The model under review builds one solid part; all positions refer to its coordinate system, in mm. Give positions to 0.01 mm unless a question says otherwise; leave off trailing zeros. Loops run counter-clockwise (first coordinate to the right, second up) from the corner with the lowest first, then second, coordinate; pieces in that order, holes last. Notation, with made-up numbers: M 20.25,-21 L 68.25,-21 A13 cw 68.25,-4 Z; hole C 77.25,-11.5 d8. An arc over 180 degrees is marked long. Return JSON: item names as keys, results as strings.
```python
from build123d import *

# Parameters (mm, degrees)
SKETCH1_W                      = 3
SKETCH1_H                      = 12.5
BOSS_EXTRUDE1_DEPTH            = 668
SKETCH2_R                      = 2
CUT_EXTRUDE1_DEPTH             = 10
CHAMFER1_SIZE                  = 2.5
LPATTERN1_COUNT                = 14
LPATTERN1_PITCH                = 50
CHAMFER1_OF_LPATTERN1_SIZE     = 2.5
LPATTERN1_COL_COUNT            = 14
LPATTERN1_COL_PITCH            = 50
CHAMFER1_OF_LPATTERN1_COL_SIZE = 2.5
CHAMFER2_SIZE                  = 1


with BuildPart() as part:
    # Sketch1 → Boss-Extrude1 (new, symmetric)
    with BuildSketch(Plane.XY):
        Rectangle(SKETCH1_W, SKETCH1_H)
    extrude(amount=BOSS_EXTRUDE1_DEPTH, both=True)

    # Sketch2 → Cut-Extrude1 (cut)
    with BuildSketch(Plane(origin=(1.5, 0, 0), x_dir=(0, 0, -1), z_dir=(1, 0, 0))):
        with Locations((0, -1.25)):
            Circle(SKETCH2_R)
    cut_extrude1 = extrude(amount=-CUT_EXTRUDE1_DEPTH, mode=Mode.SUBTRACT)

    # Chamfer1
    chamfer1_edges = [part.edges().sort_by_distance(p)[0] for p in [
        (1.5, -1.25, 2),
    ]]
    chamfer(chamfer1_edges, length=CHAMFER1_SIZE)

    # LPattern1: Cut-Extrude1 ×14
    with Locations(*[(0, 0, i * LPATTERN1_PITCH) for i in range(1, LPATTERN1_COUNT)]):
        add(cut_extrude1, mode=Mode.SUBTRACT)

    # Chamfer1 of LPattern1
    chamfer1_of_lpattern1_edges = [part.edges().sort_by_distance(p)[0] for p in [
        (1.5, -1.25, 52),
        (1.5, -1.25, 102),
        (1.5, -1.25, 152),
        (1.5, -1.25, 202),
        (1.5, -1.25, 252),
        (1.5, -1.25, 302),
        (1.5, -1.25, 352),
        (1.5, -1.25, 402),
        (1.5, -1.25, 452),
        (1.5, -1.25, 502),
        (1.5, -1.25, 552),
        (1.5, -1.25, 602),
        (1.5, -1.25, 652),
    ]]
    chamfer(chamfer1_of_lpattern1_edges, length=CHAMFER1_OF_LPATTERN1_SIZE)

    # LPattern1 col: Cut-Extrude1 ×14
    with Locations(*[(0, 0, -i * LPATTERN1_COL_PITCH) for i in range(1, LPATTERN1_COL_COUNT)]):
        add(cut_extrude1, mode=Mode.SUBTRACT)

    # Chamfer1 of LPattern1 col
    chamfer1_of_lpattern1_col_edges = [part.edges().sort_by_distance(p)[0] for p in [
        (1.5, -1.25, -48),
        (1.5, -1.25, -98),
        (1.5, -1.25, -148),
        (1.5, -1.25, -198),
        (1.5, -1.25, -248),
        (1.5, -1.25, -298),
        (1.5, -1.25, -348),
        (1.5, -1.25, -398),
        (1.5, -1.25, -448),
        (1.5, -1.25, -498),
        (1.5, -1.25, -548),
        (1.5, -1.25, -598),
        (1.5, -1.25, -648),
    ]]
    chamfer(chamfer1_of_lpattern1_col_edges, length=CHAMFER1_OF_LPATTERN1_COL_SIZE)

    # Chamfer2
    chamfer2_edges = [part.edges().sort_by_distance(p)[0] for p in [
        (-1.5, 6.25, 0),
        (1.5, 6.25, 0),
    ]]
    chamfer(chamfer2_edges, length=CHAMFER2_SIZE)


solid = part.part
```
1) Consider section A-A on z = -322.5. Write out the cut boundary in (x, y).
From the geometry:
{"outline": "M -1.5,-6.25 L 1.5,-6.25 L 1.5,5.25 L 0.5,6.25 L -0.5,6.25 L -1.5,5.25 Z"}
2) Insertion check: pin 1 (4.5 mm diameter, centred on y = -1.25, z = 550, fed in from +X); pin 2 (3 mm diameter, centred on y = -1, z = -448.5, fed in from +X); pin 3 (6.5 mm diameter, centred on y = -1.25, z = 250, fed in from +X). Each pin has a flat end and moves straight along its axis. Give the tip position at first contact, or say it passes through.
From the geometry:
{"pin 1": "x = -0.75", "pin 2": "x = 0.02", "pin 3": "x = 0.25"}
3) Wall thickness on L1, parallel to Y at x = -1.3, z = 300; L2, parallel to Y at x = -0.7, z = 569; L3, parallel to Y at x = -0.1, z = 598.5: over which ranges is each line inside the solid? List them lowest first. Write a range as from..to.
From the geometry:
{"L1": "-6.25..-3.25, 0.75..5.45", "L2": "-6.25..6.05", "L3": "-6.25..-3.73, 1.23..6.25"}
